```python
from build123d import *

# Parameters (mm, degrees)
SKETCH1_R        = 4
SKETCH1_R_2      = 1.26
EXTRUSION1_DEPTH = 4
SKETCH2_R        = 4
EXTRUSION2_DEPTH = 1
SKETCH3_R        = 4
SKETCH3_R_2      = 2.15
EXTRUSION3_DEPTH = 1


with BuildPart() as part:
    # Sketch1 → Extrusion1 (new body)
    with BuildSketch(Plane(origin=(0, 0, 0), x_dir=(-1, 0, 0), z_dir=(0, 1, 0))):
        with Locations(Location((0, 0, 0), (0, 0, 90))):
            Circle(SKETCH1_R)
        with Locations(Location((0, 0, 0), (0, 0, 90))):
            Circle(SKETCH1_R_2, mode=Mode.SUBTRACT)
    extrude(amount=EXTRUSION1_DEPTH)

    # Sketch2 → Extrusion2 (add)
    with BuildSketch(Plane(origin=(0, 4, 0), x_dir=(1, 0, 0), z_dir=(0, 1, 0))):
        with Locations(Location((0, 0, 0), (0, 0, 270))):
            Circle(SKETCH2_R)
    extrude(amount=EXTRUSION2_DEPTH)

    # Sketch3 → Extrusion3 (add)
    with BuildSketch(Plane(origin=(0, 5, 0), x_dir=(-1, 0, 0), z_dir=(0, 1, 0))):
        with Locations(Location((0, 0, 0), (0, 0, 90))):
            Circle(SKETCH3_R)
        with Locations(Location((0, 0, 0), (0, 0, 90))):
            Circle(SKETCH3_R_2, mode=Mode.SUBTRACT)
    extrude(amount=EXTRUSION3_DEPTH)


solid = part.part
```
Work out the finished part from the listing and answer in its coordinate system (mm). A direction names the side the tool comes from. Round coordinates to 2 decimals unless told otherwise and drop trailing zeros. Order: outer loops, then holes, each group sorted by start corner. A loop starts at its lowest first (then second) coordinate and runs counter-clockwise, first axis right, second up.
Q1. A tool of negligible diameter and unlimited length cuts with its end or side. For faces 1 (the flat face through (0, 5, 0)), 2 (the flat face through (1, 0, -1)), 3 (the flat face through (0, 4, 0)), from which of +Z, -Z, +X, -X, +Y, -Y can it reach the whole face along a straight path? Write none if from no direction.
Solution:
face 1: +Y
face 2: +Z, -Z, +X, -X, -Y
face 3: -Y
Q2. A cutting plane is placed at C-C, the plane y = 1.7. Determine the outline of the cut face in (x, z).
Solution:
outline: circle Ø8 at (0, 0); hole circle Ø2.52 at (0, 0)
Q3. A cutting plane is placed at B-B, the plane x = 0. Determine the outline of the cut face in (y, z), then the cut area to 3 significant figures.
Solution:
outline: (0, -4) - (6, -4) - (6, -2.15) - (5, -2.15) - (5, 2.15) - (6, 2.15) - (6, 4) - (0, 4) - (0, 1.26) - (4, 1.26) - (4, -1.26) - (0, -1.26) - close
area: 33.6 mm2
Q4. Find the intervals of material crossed by line 1 along X through (y, z) = (5.65, 0); line 2 along Y through (x, z) = (1.25, 1); line 3 along X through (y, z) = (2.9, -0.75), in increasing order.
Solution:
line 1: x = -4 to -2.15, 2.15 to 4
line 2: y = 0 to 5
line 3: x = -3.93 to -1.01, 1.01 to 3.93
Q5. The mould has two halves that part along Z. Classify faces 4 (the cylindrical face through (0.38, 1.97, 1.2)), 5 (the cylindrical face through (-3.905, 2.958, -0.867)), 6 (the flat face through (-2, 6, 2)): pulls with the +Z half, pulls with the -Z half, needs draft (parallel to the pull), parting line crosses it, or undercut.
Solution:
face 4: undercut
face 5: parting line crosses it
face 6: needs draft
Q6. A cutting plane is placed at A-A, the plane z = 0. Determine the outline of the cut face in (x, y), then the cut area to 3 significant figures.
Solution:
outline: (-4, 0) - (-1.26, 0) - (-1.26, 4) - (1.26, 4) - (1.26, 0) - (4, 0) - (4, 6) - (2.15, 6) - (2.15, 5) - (-2.15, 5) - (-2.15, 6) - (-4, 6) - close
area: 33.6 mm2
Q7. A cutting plane is placed at D-D, the plane y = 4.8. Determine the outline of the cut face in (x, z), then the cut area to 3 significant figures.
Solution:
outline: circle Ø8 at (0, 0)
area: 50.3 mm2
